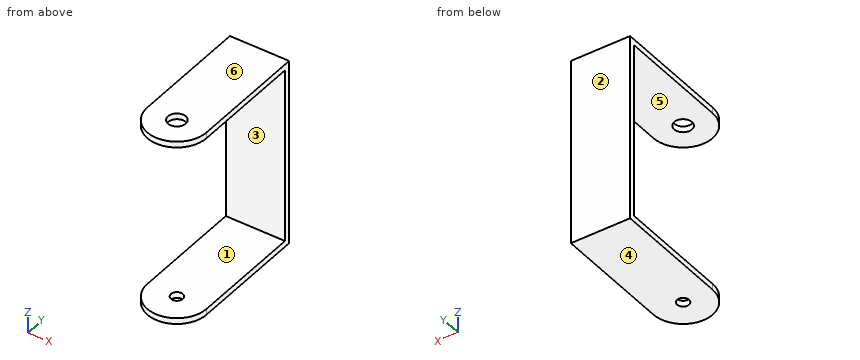
```python
from build123d import *

# Parameters (mm, degrees)
EXTRUDE_1_DEPTH     = 2
SKETCH_2_W          = 20
SKETCH_2_H          = 2
EXTRUDE_2_DEPTH     = 61.3
CUT_EXTRUDE_1_REACH = 79.504
SKETCH_4_R          = 3
SKETCH_6_R          = 2
CUT_EXTRUDE_2_DEPTH = 2


with BuildPart() as part:
    # 草图1 → 凸台-拉伸1 (new body)
    with BuildSketch(Plane.XY):
        with BuildLine():
            Line((0, 0), (0, 40))
            Line((0, 40), (20, 40))
            Line((20, 40), (20, 0))
            ThreePointArc((20, 0), (10, -10), (0, 0))
        make_face()
    extrude_1 = extrude(amount=EXTRUDE_1_DEPTH)

    # 草图2 → 凸台-拉伸2 (add)
    with BuildSketch(Plane.XY.offset(2)):
        with Locations((10, 39)):
            Rectangle(SKETCH_2_W, SKETCH_2_H)
    extrude(amount=EXTRUDE_2_DEPTH)

    # 镜向1: 凸台-拉伸1 across plane
    add(extrude_1.mirror(Plane.XY.offset(31.65)))

    # 草图4 → 切除-拉伸1 (cut, up to next)
    with BuildSketch(Plane.XY.offset(63.3), mode=Mode.PRIVATE) as cut_extrude_1_sk1:
        with Locations((10, 0)):
            Circle(SKETCH_4_R)
    cut_extrude_1_tool1 = extrude(cut_extrude_1_sk1.sketch, amount=-CUT_EXTRUDE_1_REACH, mode=Mode.PRIVATE) & part.part
    add(cut_extrude_1_tool1.solids().sort_by_distance((10, 0, 63.3))[0], mode=Mode.SUBTRACT)

    # 草图6 → 切除-拉伸2 (cut)
    with BuildSketch(Plane.XY.offset(2)):
        with Locations((10, 0)):
            Circle(SKETCH_6_R)
    extrude(amount=-CUT_EXTRUDE_2_DEPTH, mode=Mode.SUBTRACT)


solid = part.part
```
Can you work these out from the model? Positions are in its coordinate system, mm. Face numbers are marked on the shaded views. A direction names the side the tool comes from. Give positions to 0.01 mm unless a question says otherwise; leave off trailing zeros. Write each loop counter-clockwise with the first axis right and the second up, starting at its lowest first coordinate (ties: lowest second). Pieces come first, ordered by that corner, then holes. Notation, with made-up numbers: (21.25, 74.25) - (68.25, 74.25) arc R15 ccw to (68.25, 90.25) - close; hole circle Ø3 at (-28, -7). An arc over 180 degrees is marked (long way). Write item = value, one per line. Start each with the question number.
1. Imagine slicing it at C-C (x = 16.25). Please give me the cut outline in (y, z), and give its area (3 significant figures).
2. Imagine slicing it at B-B (x = 10). Please give me the cut outline in (y, z).
3. On a 3-axis mill with a long thin cutter (end or side, diameter ignored), from which of +Z, -Z, +X, -X, +Y, -Y can I reach the whole of each face in a straight line? I mean the marked faces 5 and 6. Say none if no direction works.
4. Imagine slicing it at D-D (z = 32). Please give me the cut outline in (x, y), and give its area (3 significant figures).
5. Thinking about a two-plate mould opening in Z: for the marked faces 1, 2, 3 and 4, which applies, released by +Z, released by -Z, zero draft, split by the parting line, or undercut?
6. For pin 1 (10 mm diameter, centred on x = 10.5, z = 27, fed in from -Y); pin 2 (9.5 mm diameter, centred on x = 10, y = 0, fed in from -Z); pin 3 (3.5 mm diameter, centred on x = 10, y = 0, fed in from -Z), each with a flat end and sliding along its axis, tell me the tip position at first contact or that it passes through.
7. Please list where these lines run through material, in increasing order: line 1 (Y direction, x = 10, z = 1); line 2 (Z direction, x = 16.5, y = 34.5); line 3 (Y direction, x = 10, z = 62.1).
8. Imagine slicing it at A-A (y = 4.5). Please give me the cut outline in (x, z).
Worked answers:
q1.outline = (-7.81, 0) - (40, 0) - (40, 63.3) - (-7.81, 63.3) - (-7.81, 61.3) - (38, 61.3) - (38, 2) - (-7.81, 2) - close
q1.area = 310 mm2
q2.outline = (-10, 0) - (-2, 0) - (-2, 2) - (-10, 2) - close; (-10, 61.3) - (-3, 61.3) - (-3, 63.3) - (-10, 63.3) - close; (2, 0) - (40, 0) - (40, 63.3) - (3, 63.3) - (3, 61.3) - (38, 61.3) - (38, 2) - (2, 2) - close
q3.face_5 = +X, -X, -Y
q3.face_6 = +Z, +X, -X, +Y, -Y
q4.outline = (0, 38) - (20, 38) - (20, 40) - (0, 40) - close
q4.area = 40.0 mm2
q5.face_1 = undercut
q5.face_2 = zero draft
q5.face_3 = undercut
q5.face_4 = released by -Z
q6.pin_1 = 38
q6.pin_2 = 0
q6.pin_3 = through
q7.line_1 = -10 to -2, 2 to 40
q7.line_2 = 0 to 2, 61.3 to 63.3
q7.line_3 = -10 to -3, 3 to 40
q8.outline = (0, 0) - (20, 0) - (20, 2) - (0, 2) - close; (0, 61.3) - (20, 61.3) - (20, 63.3) - (0, 63.3) - close
